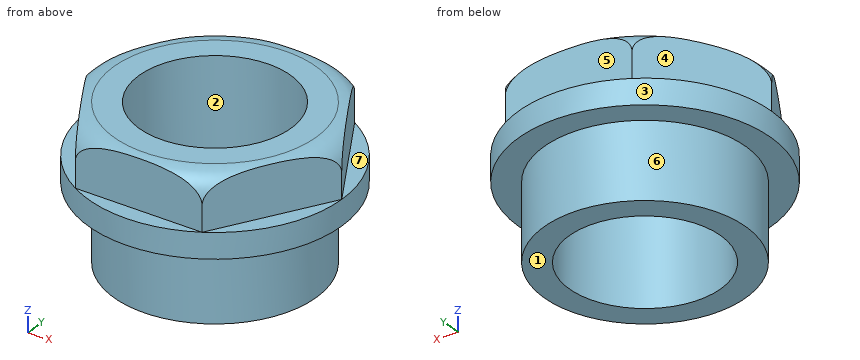
```python
from build123d import *

# Parameters (mm, degrees)
SKETCH_1_R          = 8
EXTRUDE_1_DEPTH     = 6
SKETCH_2_R          = 10
EXTRUDE_2_DEPTH     = 6
FILLET_1_R          = 2
SKETCH_3_OUTSIDE_W  = 28.144
SKETCH_3_OUTSIDE_H  = 28.144
CUT_EXTRUDE_1_DEPTH = 4
SKETCH_4_R          = 6
CUT_EXTRUDE_2_DEPTH = 12


with BuildPart() as part:
    # 草图1 → 凸台-拉伸1 (new body)
    with BuildSketch(Plane.XY):
        Circle(SKETCH_1_R)
    extrude(amount=EXTRUDE_1_DEPTH)

    # 草图2 → 凸台-拉伸2 (add)
    with BuildSketch(Plane.XY.offset(6)):
        Circle(SKETCH_2_R)
    extrude(amount=EXTRUDE_2_DEPTH)

    # 圆角1
    fillet_1_edges = [part.edges().sort_by_distance(p)[0] for p in [
        (-10, 0, 12),
    ]]
    fillet(fillet_1_edges, radius=FILLET_1_R)

    # 草图3 outside → 切除-拉伸1 (cut)
    with BuildSketch(Plane.XY.offset(12)):
        Rectangle(SKETCH_3_OUTSIDE_W, SKETCH_3_OUTSIDE_H)
        Polygon((10, 0), (5, 8.660254038), (-5, 8.660254038), (-10, 0), (-5, -8.660254038), (5, -8.660254038), align=None, mode=Mode.SUBTRACT)
    extrude(amount=-CUT_EXTRUDE_1_DEPTH, mode=Mode.SUBTRACT)

    # 草图4 → 切除-拉伸2 (cut)
    with BuildSketch(Plane(origin=(0, 0, 0), x_dir=(-1, 0, 0), z_dir=(0, 0, -1))):
        Circle(SKETCH_4_R)
    extrude(amount=-CUT_EXTRUDE_2_DEPTH, mode=Mode.SUBTRACT)


solid = part.part
```
Check sheet for the modelled part. Datum: model origin and axes. Units: mm. Face numbers are marked on the shaded views. A direction names the side the tool comes from. Give positions to 0.01 mm unless a question says otherwise; leave off trailing zeros. Write each loop counter-clockwise with the first axis right and the second up, starting at its lowest first coordinate (ties: lowest second). Pieces come first, ordered by that corner, then holes. Notation, with made-up numbers: (32, 33.25) - (74, 33.25) arc R8 ccw to (74, 42.25) - close; hole circle Ø7 at (-27.75, 56.25). An arc over 180 degrees is marked (long way). Answer as a JSON object with one key per item and string values. Group by question number.
1) Sectioned sample at D-D (z = 6.5). Record the cut outline in (x, y).
2) Sectioned sample at B-B (z = 9.5). Record the cut outline in (x, y).
3) Access from +Z, -Z, +X, -X, +Y, -Y to the whole of each face (thin tool, end or side, straight path). Record for the marked faces 5, 6 and 7.
4) Release check for a two-part mould opening along Y. For the marked faces 1, 2, 3 and 4 record: pulls with the +Y half, pulls with the -Y half, needs draft (parallel to the pull), parting line crosses it, or undercut.
5) Depth check by flat-ended pin: P1, Ø1.2, axis at x = -1, z = 11, coming from the -Y side; P2, Ø1.9, axis at x = 2.5, z = 10.5, coming from the +Y side; P3, Ø1.5, axis at x = 8, y = -6.5, coming from the +Z side. Enter the tip coordinate at first touch or a pass-through.
6) Thickness scan on probe 1 along Y at (x, z) = (0, 8.25); probe 2 along Y at (x, z) = (0, 5.75); probe 3 along X at (y, z) = (1, 4.25). Record the ranges inside material, lowest first. Write a range as from..to.
7) Sectioned sample at C-C (z = 5.25). Record the cut outline in (x, y).
8) Sectioned sample at A-A (x = 0). Record the cut outline in (y, z), then the cut area to 3 significant figures.
Geometry results:
{
 "1": {"outline": "circle Ø20 at (0, 0); hole circle Ø12 at (0, 0)"},
 "2": {"outline": "(-10, 0) - (-5, -8.66) - (5, -8.66) - (10, 0) - (5, 8.66) - (-5, 8.66) - close; hole circle Ø12 at (0, 0)"},
 "3": {"face 5": "+Z, +X, -X, +Y", "face 6": "-Z", "face 7": "+Z, +X, +Y"},
 "4": {"face 1": "needs draft", "face 2": "undercut", "face 3": "parting line crosses it", "face 4": "pulls with the +Y half"},
 "5": {"P1": "stops at y = -8.66", "P2": "stops at y = 8.66", "P3": "stops at z = 8"},
 "6": {"probe 1": "y = -8.66..-6, 6..8.66", "probe 2": "y = -8..-6, 6..8", "probe 3": "x = -7.94..-5.92, 5.92..7.94"},
 "7": {"outline": "circle Ø16 at (0, 0); hole circle Ø12 at (0, 0)"},
 "8": {"outline": "(-10, 6) - (-8, 6) - (-8, 0) - (-6, 0) - (-6, 12) - (-8, 12) arc R2 ccw to (-8.66, 11.89) - (-8.66, 8) - (-10, 8) - close; (6, 0) - (8, 0) - (8, 6) - (10, 6) - (10, 8) - (8.66, 8) - (8.66, 11.89) arc R2 ccw to (8, 12) - (6, 12) - close", "area": "61.2 mm^2"}
}
